from build123d import *

# Parameters (mm, degrees)
F0_W     = 50.8
F0_H     = 228.6
F1_DEPTH = 25.4
F2_W     = 47.5996
F2_H     = 22.1996
F3_DEPTH = 228.601
F5_D     = 5.1054
F7_D     = 5.1054


with BuildPart() as f1:
    # F0 (on Top) → F1 (new body)
    with BuildSketch(Plane.XY):
        with Locations((-77.71441, 39.378307)):
            Rectangle(F0_W, F0_H)
    extrude(amount=F1_DEPTH)

    # F2 (on face) → F3 (cut, through all)
    with BuildSketch(Plane(origin=(0, 153.678307, 0), x_dir=(-1, 0, 0), z_dir=(0, 1, 0))):
        with Locations((77.71441, 12.7)):
            Rectangle(F2_W, F2_H)
    extrude(amount=-F3_DEPTH, mode=Mode.SUBTRACT)

    # F5 (through all)
    with Locations(Plane.XY.offset(25.4)):
        with Locations((-65.01441, 39.378307), (-65.01441, -36.821693), (-65.01441, 13.978307), (-65.01441, 115.578307), (-65.01441, 90.178307), (-65.01441, 140.978307), (-65.01441, 64.778307), (-90.41441, 140.978307), (-90.41441, 115.578307), (-90.41441, 90.178307), (-90.41441, 64.778307), (-90.41441, 39.378307), (-90.41441, 13.978307), (-90.41441, -11.421693), (-90.41441, -36.821693), (-65.01441, -62.221693), (-90.41441, -62.221693), (-65.01441, -11.421693)):
            Hole(F5_D / 2)

    # F7 (through all)
    with Locations(Plane(origin=(-103.11441, 0, 0), x_dir=(0, -1, 0), z_dir=(-1, 0, 0))):
        with Locations((-140.978307, 12.7), (-90.178307, 12.7), (-115.578307, 12.7), (-39.378307, 12.7), (-64.778307, 12.7), (11.421693, 12.7), (-13.978307, 12.7), (62.221693, 12.7), (36.821693, 12.7)):
            Hole(F7_D / 2)


solid = f1.part
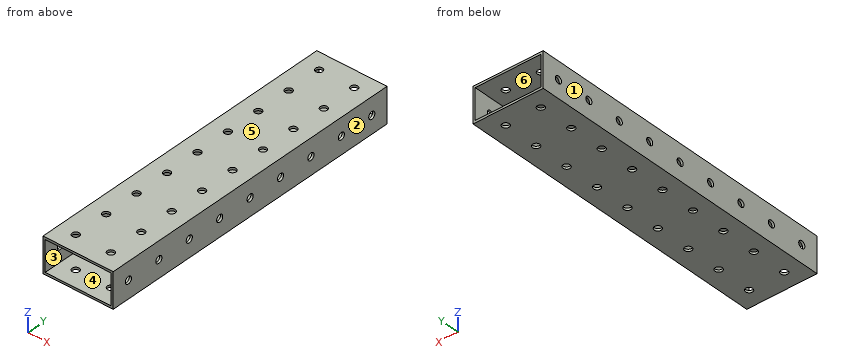
The listing builds one solid part. Answer for the finished solid, in the listing's coordinates (mm). Face numbers are marked on the shaded views. A direction names the side the tool comes from. Coordinates: 2 decimals unless noted, no trailing zeros. Write each loop counter-clockwise with the first axis right and the second up, starting at its lowest first coordinate (ties: lowest second). Pieces come first, ordered by that corner, then holes. Notation, with made-up numbers: (37.25, -3.5) - (76.25, -3.5) arc R24 cw to (76.25, 27.5) - close; hole circle Ø4 at (-20, 10.5). An arc over 180 degrees is marked (long way). Answer as CSV lines item,"result".
1. Determine the mould class of the marked faces 1, 2, 3 and 4 for opening direction X: +X half, -X half, draft (parallel to the pull), parting line (faces both ways), or undercut.
Computed values:
face 1,"-X half"
face 2,"+X half"
face 3,"undercut"
face 4,"undercut"
2. Straight lines are drawn through the part: line 1 (Z direction, x = -61.5, y = 37.5); line 2 (X direction, y = 27, z = 2.5). For each, find the intervals that lie inside material, in ascending order. Write a range as [from, to].
Computed values:
line 1,"z = [0, 1.6], [23.8, 25.4]"
line 2,"x = [-103.11, -101.51], [-53.91, -52.31]"
3. A tool of negligible diameter and unlimited length cuts with its end or side. For the marked faces 5 and 6, from which of +Z, -Z, +X, -X, +Y, -Y can it reach the whole face along a straight path? Write none if from no direction.
Computed values:
face 5,"+Z, +X, -X, +Y, -Y"
face 6,"+Y, -Y"
4. Find section D-D (z = 12.7). Give the number of separate pieces and of enclosed holes in the cut face, plus the area to 3 significant figures.
Computed values:
separate pieces,"20"
enclosed holes,"0"
area,"585 mm²"
5. Find section A-A (x = -81). Give the vertices of the cut face in (y, z), plus the area to 3 significant figures.
Computed values:
outline,"(-74.92, 0) - (153.68, 0) - (153.68, 1.6) - (-74.92, 1.6) - close; (-74.92, 23.8) - (153.68, 23.8) - (153.68, 25.4) - (-74.92, 25.4) - close"
area,"732 mm²"
6. Find section C-C (y = 70.5). Give the vertices of the cut face in (x, z).
Computed values:
outline,"(-103.11, 0) - (-52.31, 0) - (-52.31, 25.4) - (-103.11, 25.4) - close; hole (-101.51, 1.6) - (-53.91, 1.6) - (-53.91, 23.8) - (-101.51, 23.8) - close"
7. Find section B-B (z = 21). Give the vertices of the cut face in (x, y).
Computed values:
outline,"(-103.11, -74.92) - (-101.51, -74.92) - (-101.51, 153.68) - (-103.11, 153.68) - close; (-53.91, -74.92) - (-52.31, -74.92) - (-52.31, 153.68) - (-53.91, 153.68) - close"
